Read the model definition and answer for the solid it produces. Units are mm, in the model's axes. A direction names the side the tool comes from. Coordinates: 2 decimals unless noted, no trailing zeros. Order: outer loops, then holes, each group sorted by start corner. A loop starts at its lowest first (then second) coordinate and runs counter-clockwise, first axis right, second up. Notation, with made-up numbers: (8, -3) -> (51, -3) arc R21 cw to (51, 27) -> close; hole circle Ø1 at (28, 59.5). An arc over 180 degrees is marked (long way). Use CSV: the item, a comma, the result in double quotes.
```python
from build123d import *

# Parameters (mm, degrees)
CROQUIS1_W              = 77
CROQUIS1_H              = 45
SALIENTE_EXTRUIR1_DEPTH = 3
CORTAR_EXTRUIR1_REACH   = 5
CROQUIS2_R              = 1.6
CROQUIS2_W              = 12.1
CROQUIS2_H              = 10.65
CROQUIS2_H_2            = 9.15


with BuildPart() as part:
    # Croquis1 → Saliente-Extruir1 (new body)
    with BuildSketch(Plane.XY):
        Rectangle(CROQUIS1_W, CROQUIS1_H)
    extrude(amount=SALIENTE_EXTRUIR1_DEPTH)

    # Croquis2 → Cortar-Extruir1 (cut, up to next)
    with BuildSketch(Plane(origin=(0, 0, 0), x_dir=(-1, 0, 0), z_dir=(0, 0, -1)), mode=Mode.PRIVATE) as cortar_extruir1_sk1:
        with Locations((34.75, 17.5)):
            Circle(CROQUIS2_R)
    cortar_extruir1_tool1 = extrude(cortar_extruir1_sk1.sketch, amount=-CORTAR_EXTRUIR1_REACH, mode=Mode.PRIVATE) & part.part
    add(cortar_extruir1_tool1.solids().sort_by_distance((-34.75, 17.5, 0))[0], mode=Mode.SUBTRACT)
    # Croquis2 → Cortar-Extruir1 (cut, up to next)
    with BuildSketch(Plane(origin=(0, 0, 0), x_dir=(-1, 0, 0), z_dir=(0, 0, -1)), mode=Mode.PRIVATE) as cortar_extruir1_sk2:
        with Locations((-34.75, 17.5)):
            Circle(CROQUIS2_R)
    cortar_extruir1_tool2 = extrude(cortar_extruir1_sk2.sketch, amount=-CORTAR_EXTRUIR1_REACH, mode=Mode.PRIVATE) & part.part
    add(cortar_extruir1_tool2.solids().sort_by_distance((34.75, 17.5, 0))[0], mode=Mode.SUBTRACT)
    # Croquis2 → Cortar-Extruir1 (cut, up to next)
    with BuildSketch(Plane(origin=(0, 0, 0), x_dir=(-1, 0, 0), z_dir=(0, 0, -1)), mode=Mode.PRIVATE) as cortar_extruir1_sk3:
        with Locations((-34.75, -17.5)):
            Circle(CROQUIS2_R)
    cortar_extruir1_tool3 = extrude(cortar_extruir1_sk3.sketch, amount=-CORTAR_EXTRUIR1_REACH, mode=Mode.PRIVATE) & part.part
    add(cortar_extruir1_tool3.solids().sort_by_distance((34.75, -17.5, 0))[0], mode=Mode.SUBTRACT)
    # Croquis2 → Cortar-Extruir1 (cut, up to next)
    with BuildSketch(Plane(origin=(0, 0, 0), x_dir=(-1, 0, 0), z_dir=(0, 0, -1)), mode=Mode.PRIVATE) as cortar_extruir1_sk4:
        with Locations((34.75, -17.5)):
            Circle(CROQUIS2_R)
    cortar_extruir1_tool4 = extrude(cortar_extruir1_sk4.sketch, amount=-CORTAR_EXTRUIR1_REACH, mode=Mode.PRIVATE) & part.part
    add(cortar_extruir1_tool4.solids().sort_by_distance((-34.75, -17.5, 0))[0], mode=Mode.SUBTRACT)
    # Croquis2 → Cortar-Extruir1 (cut, up to next)
    with BuildSketch(Plane(origin=(0, 0, 0), x_dir=(-1, 0, 0), z_dir=(0, 0, -1)), mode=Mode.PRIVATE) as cortar_extruir1_sk5:
        with Locations((20, 9.675)):
            Rectangle(CROQUIS2_W, CROQUIS2_H)
    cortar_extruir1_tool5 = extrude(cortar_extruir1_sk5.sketch, amount=-CORTAR_EXTRUIR1_REACH, mode=Mode.PRIVATE) & part.part
    add(cortar_extruir1_tool5.solids().sort_by_distance((-20, 9.675, 0))[0], mode=Mode.SUBTRACT)
    # Croquis2 → Cortar-Extruir1 (cut, up to next)
    with BuildSketch(Plane(origin=(0, 0, 0), x_dir=(-1, 0, 0), z_dir=(0, 0, -1)), mode=Mode.PRIVATE) as cortar_extruir1_sk6:
        with Locations((20, -10.125)):
            Rectangle(CROQUIS2_W, CROQUIS2_H_2)
    cortar_extruir1_tool6 = extrude(cortar_extruir1_sk6.sketch, amount=-CORTAR_EXTRUIR1_REACH, mode=Mode.PRIVATE) & part.part
    add(cortar_extruir1_tool6.solids().sort_by_distance((-20, -10.125, 0))[0], mode=Mode.SUBTRACT)


solid = part.part
```
Item 1: A tool of negligible diameter and unlimited length cuts with its end or side. For faces 5 (the flat face through (-20, 4.35, 1)), 6 (the flat face through (38.5, 0, 1)), from which of +Z, -Z, +X, -X, +Y, -Y can it reach the whole face along a straight path? Write none if from no direction.
Return value:
face 5,"+Z, -Z"
face 6,"+Z, -Z, +X, +Y, -Y"
Item 2: The mould has two halves that part along Y. Classify faces 1 (the flat face through (-38.5, 0, 1)), 2 (the flat face through (-1, -22.5, 1)), 3 (the flat face through (-1, 22.5, 1)), 4 (the flat face through (-20, -14.7, 1)): +Y half, -Y half, draft (parallel to the pull), parting line (faces both ways), or undercut.
Return value:
face 1,"draft"
face 2,"-Y half"
face 3,"+Y half"
face 4,"undercut"
Item 3: Find section B-B, the plane y = -9. Give the vertices of the cut face in (x, z).
Return value:
outline,"(-38.5, 0) -> (-26.05, 0) -> (-26.05, 3) -> (-38.5, 3) -> close; (-13.95, 0) -> (38.5, 0) -> (38.5, 3) -> (-13.95, 3) -> close"
Item 4: Find section A-A, the plane x = 34.75. Give the vertices of the cut face in (y, z).
Return value:
outline,"(-22.5, 0) -> (-19.1, 0) -> (-19.1, 3) -> (-22.5, 3) -> close; (-15.9, 0) -> (15.9, 0) -> (15.9, 3) -> (-15.9, 3) -> close; (19.1, 0) -> (22.5, 0) -> (22.5, 3) -> (19.1, 3) -> close"
Item 5: Find section C-C, the plane z = 0.7. Give the vertices of the cut face in (x, y), then the cut area to 3 significant figures.
Return value:
outline,"(-38.5, -22.5) -> (38.5, -22.5) -> (38.5, 22.5) -> (-38.5, 22.5) -> close; hole circle Ø3.2 at (-34.75, -17.5); hole circle Ø3.2 at (-34.75, 17.5); hole (-26.05, -14.7) -> (-13.95, -14.7) -> (-13.95, -5.55) -> (-26.05, -5.55) -> close; hole (-26.05, 4.35) -> (-13.95, 4.35) -> (-13.95, 15) -> (-26.05, 15) -> close; hole circle Ø3.2 at (34.75, -17.5); hole circle Ø3.2 at (34.75, 17.5)"
area,"3,190 mm^2"
Item 6: Straight lines are drawn through the part: line 1 along Y through (x, z) = (-34.75, 1.8); line 2 along Y through (x, z) = (-20, 0.95); line 3 along X through (y, z) = (-11.5, 0.45). For each, find the intervals that lie inside material, in ascending order.
Return value:
line 1,"y = -22.5 to -19.1, -15.9 to 15.9, 19.1 to 22.5"
line 2,"y = -22.5 to -14.7, -5.55 to 4.35, 15 to 22.5"
line 3,"x = -38.5 to -26.05, -13.95 to 38.5"
Item 7: Find section D-D, the plane y = 17.5. Give the vertices of the cut face in (x, z).
Return value:
outline,"(-38.5, 0) -> (-36.35, 0) -> (-36.35, 3) -> (-38.5, 3) -> close; (-33.15, 0) -> (33.15, 0) -> (33.15, 3) -> (-33.15, 3) -> close; (36.35, 0) -> (38.5, 0) -> (38.5, 3) -> (36.35, 3) -> close"
